```python
from build123d import *

# Parameters (mm, degrees)
SKETCH_1_R          = 3.61
EXTRUDE_1_DEPTH     = 4
CUT_EXTRUDE_1_DEPTH = 2
SKETCH_3_R          = 2
EXTRUDE_2_DEPTH     = 12


with BuildPart() as part:
    # Sketch 1 → Extrude 1 (new body)
    with BuildSketch(Plane(origin=(0, 0, 0), x_dir=(1, 0, 0), z_dir=(0, 1, 0))):
        with Locations(Location((0, 0, 0), (0, 0, 270))):
            Circle(SKETCH_1_R)
    extrude(amount=EXTRUDE_1_DEPTH)

    # Sketch 2 → Cut-Extrude 1 (cut)
    with BuildSketch(Plane.XZ):
        Polygon((1.732050808, 0), (0.866025404, 1.5), (-0.866025404, 1.5), (-1.732050808, 0), (-0.866025404, -1.5), (0.866025404, -1.5), align=None)
    extrude(amount=-CUT_EXTRUDE_1_DEPTH, mode=Mode.SUBTRACT)

    # Sketch 3 → Extrude 2 (add)
    with BuildSketch(Plane(origin=(0, 4, 0), x_dir=(1, 0, 0), z_dir=(0, 1, 0))):
        with Locations(Location((0, 0, 0), (0, 0, 270))):
            Circle(SKETCH_3_R)
    extrude(amount=EXTRUDE_2_DEPTH)


solid = part.part
```
Work out the finished part from the listing and answer in its coordinate system (mm). A direction names the side the tool comes from. Give positions to 0.01 mm unless a question says otherwise; leave off trailing zeros. Order: outer loops, then holes, each group sorted by start corner. A loop starts at its lowest first (then second) coordinate and runs counter-clockwise, first axis right, second up. Notation, with made-up numbers: (53.5, 27.5) -> (75.5, 27.5) arc R7 cw to (75.5, 35.5) -> close; hole circle Ø10 at (10.25, 88). An arc over 180 degrees is marked (long way). Answer as CSV lines item,"result". Start each with the question number.
(1) Each of these flat-tipped pins is pushed along its axis until it touches: pin 1 Ø3 at (x, y) = (-1.5, 6) entering from +Z; pin 2 Ø1.5 at (x, y) = (-2.5, 12) entering from +Z; pin 3 Ø3 at (y, z) = (11.5, 2) entering from +X. Where does it stop, or does it pass through?
(2) Section A-A, the plane x = 0 is taken. Write down the section's boundary in (y, z), plus the area to 3 significant figures.
(3) Which of the six approach directions +Z, -Z, +X, -X, +Y, -Y give full straight-line access (tool end or side, diameter ignored) to faces 1 (the flat face through (-1.293, 0.986, 0.76)), 2 (the flat face through (0, 0, 2)), 3 (the flat face through (-2, 4, 2))?
(4) Consider line 1 along Y through (x, z) = (-1.25, 0); line 2 along X through (y, z) = (6, 0); line 3 along Y through (x, z) = (0, 3). Determine where each line is inside the solid, lowest interval first.
(5) Section C-C, the plane z = 1 is taken. Write down the section's boundary in (x, y), plus the area to 3 significant figures.
(6) Section B-B, the plane y = 14.5 is taken. Write down the section's boundary in (x, z), plus the area to 3 significant figures.
(7) Section D-D, the plane z = -2.5 is taken. Write down the section's boundary in (x, y).
(8) For a pull along X with two mould halves and no side action, classify faces 4 (the cylindrical face through (-2, 10, 0)), 5 (the flat face through (0, 2, 0)), 6 (the flat face through (0, 1, 1.5)), 7 (the flat face through (0, 16, 0)) as released by +X, released by -X, zero draft, split by the parting line, or undercut.
Entries:
1,pin 1,"z = 2"
1,pin 2,"z = 0.97"
1,pin 3,"x = 1.94"
2,outline,"(0, -3.61) -> (4, -3.61) -> (4, -2) -> (16, -2) -> (16, 2) -> (4, 2) -> (4, 3.61) -> (0, 3.61) -> (0, 1.5) -> (2, 1.5) -> (2, -1.5) -> (0, -1.5) -> close"
2,area,"70.9 mm²"
3,face 1,"-Y"
3,face 2,"+Z, -Z, +X, -X, -Y"
3,face 3,"+Y"
4,line 1,"2 to 16"
4,line 2,"-2 to 2"
4,line 3,"0 to 4"
5,outline,"(-3.47, 0) -> (-1.15, 0) -> (-1.15, 2) -> (1.15, 2) -> (1.15, 0) -> (3.47, 0) -> (3.47, 4) -> (1.73, 4) -> (1.73, 16) -> (-1.73, 16) -> (-1.73, 4) -> (-3.47, 4) -> close"
5,area,"64.7 mm²"
6,outline,"circle Ø4 at (0, 0)"
6,area,"12.6 mm²"
7,outline,"(-2.6, 0) -> (2.6, 0) -> (2.6, 4) -> (-2.6, 4) -> close"
8,face 4,"split by the parting line"
8,face 5,"undercut"
8,face 6,"undercut"
8,face 7,"zero draft"
